Job drawing, mm, ordinate dimensions from the low corner. One solid piece. Give positions to 0.01 mm unless a question says otherwise; leave off trailing zeros. Write each loop counter-clockwise with the first axis right and the second up, starting at its lowest first coordinate (ties: lowest second). Pieces come first, ordered by that corner, then holes. Notation, with made-up numbers: (14, 81.5) - (36, 81.5) arc R34 ccw to (36, 120.5) - close; hole circle Ø2 at (31.5, -1.75). An arc over 180 degrees is marked (long way). Put each result on its own line as item: value. Start each with the question number.
1. Wall check: line 1 (X direction, y = 11.75, z = 4.25) (1 decimal); line 2 (Z direction, x = 4.5, y = 5.25) (1 decimal); line 3 (Z direction, x = 8.5, y = 6.5) (1 decimal). Give the ranges that are in metal, low to high.
2. Mould opens along X. For the marked faces 1, 2, 3 and 4 say: +X half, -X half, draft (parallel to the pull), parting line (faces both ways), or undercut.
3. Drop flat-ended pins along their axis: pin 1 (2 mm diameter, centred on x = 4, y = 8.5, fed in from -Z); pin 2 (3 mm diameter, centred on y = 2.5, z = 9, fed in from +X); pin 3 (1 mm diameter, centred on x = 8.5, y = 4, fed in from +Z). Give the stop position or say it passes through.
4. Cut at A-A on y = 14.25. List the corners of the cut face in (x, z) (1 decimal).
5. Cut at B-B on y = 9. List the corners of the cut face in (x, z) (1 decimal).
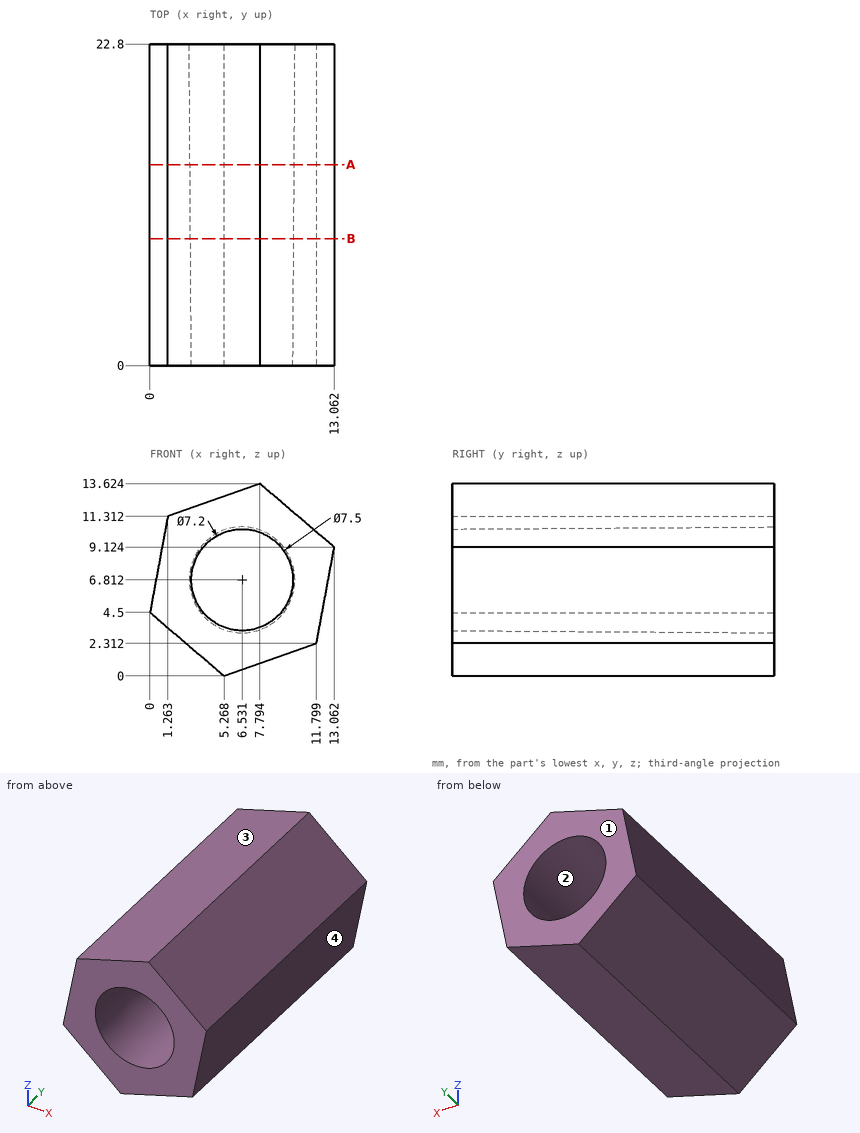
Report:
1. line 1: x = 0.3 to 3.9, 9.2 to 12.2
1. line 2: z = 0.7 to 3.8, 9.8 to 12.5
1. line 3: z = 1.1 to 3.7, 9.9 to 13
2. face 1: draft
2. face 2: undercut
2. face 3: -X half
2. face 4: +X half
3. pin 1: stops at z = 0.23
3. pin 2: stops at x = 13.06
3. pin 3: stops at z = 13.45
4. outline: (0, 4.5) - (5.3, 0) - (11.8, 2.3) - (13.1, 9.1) - (7.8, 13.6) - (1.3, 11.3) - close; hole circle Ø7.4 at (6.5, 6.8)
5. outline: (0, 4.5) - (5.3, 0) - (11.8, 2.3) - (13.1, 9.1) - (7.8, 13.6) - (1.3, 11.3) - close; hole circle Ø7.3 at (6.5, 6.8)
